Source: three-view drawing plus pictorial views. Frame: mm from the lowest corner of the part. Give positions to 0.01 mm unless a question says otherwise; leave off trailing zeros. Loops run counter-clockwise (first coordinate to the right, second up) from the corner with the lowest first, then second, coordinate; pieces in that order, holes last. Notation, with made-up numbers: (84, 0.25) -> (142, 0.25) arc R16 cw to (142, 23.25) -> close; hole circle Ø5 at (60, 34.25). An arc over 180 degrees is marked (long way). Put each result on its own line as item: value.
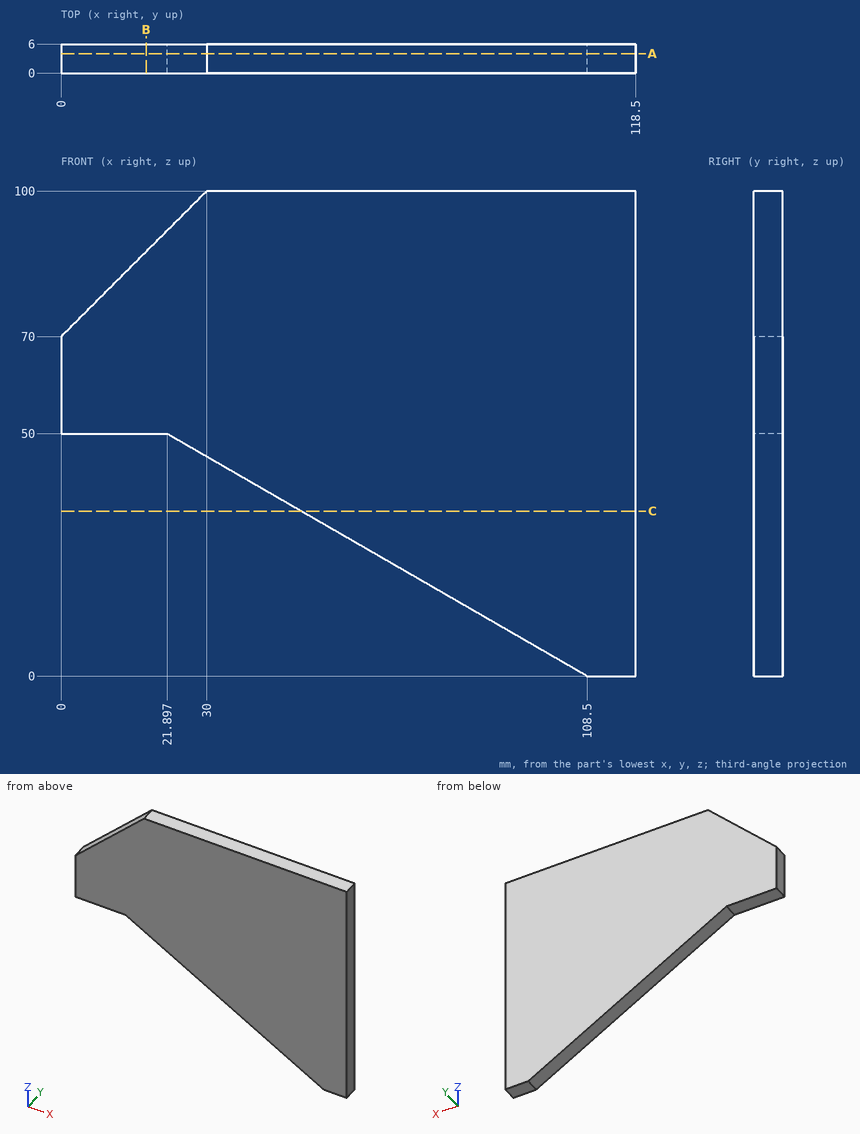
(1) Section A-A on y = 4. Return loops of the section in (x, z), then the cut area to 3 significant figures.
Calculated:
outline: (0, 50) -> (21.9, 50) -> (108.5, 0) -> (118.5, 0) -> (118.5, 100) -> (30, 100) -> (0, 70) -> close
area: 8,140 mm²
(2) First-contact query: P1, Ø3, axis at x = 10, y = 2, coming from the -Z side; P2, Ø3, axis at x = 29.5, y = 4, coming from the -Z side (1 decimal). Flat tips, straight axial feed; report the tip coordinate or a pass-through.
Calculated:
P1: stops at z = 50
P2: stops at z = 44.7
(3) Line query: probe 1 along Z at (x, y) = (56.5, 1.5); probe 2 along Z at (x, y) = (31.5, 2) (1 decimal); probe 3 along X at (y, z) = (2.75, 86). Output: solid intervals per line, ascending. Write a range as from..to.
Calculated:
probe 1: z = 30.02..100
probe 2: z = 44.5..100
probe 3: x = 16..118.5
(4) Section B-B on x = 17.5. Return loops of the section in (y, z).
Calculated:
outline: (0, 50) -> (6, 50) -> (6, 87.5) -> (0, 87.5) -> close
(5) Section C-C on z = 34. Return loops of the section in (x, y), then the cut area to 3 significant figures.
Calculated:
outline: (49.61, 0) -> (118.5, 0) -> (118.5, 6) -> (49.61, 6) -> close
area: 413 mm²
